```python
from build123d import *

# Parameters (mm, degrees)
MAIN_SKETCH_W        = 110
MAIN_SKETCH_H        = 72
MAIN_EXTRUSION_DEPTH = 6
MAIN_HOLE_SKETCH_R   = 1
MAIN_HOLE_SKETCH_R_2 = 0.9
MAIN_HOLE_DEPTH      = 7
EPIA_FIX_SKETCH_W    = 77
EPIA_FIX_SKETCH_H    = 40
EPIA_FIX_SKETCH_W_2  = 15
EPIA_FIX_SKETCH_H_2  = 8
EPIA_FIX_SKETCH_W_3  = 10
EPIA_FIX_SKETCH_W_4  = 8
EPIA_FIX_SKETCH_H_3  = 16
EPIA_FIX_DEPTH       = 4
FIX_SKETCH_R         = 1.35
FIX_HOLE_DEPTH       = 7


with BuildPart() as part:
    # Main-Sketch → Main-Extrusion (new body)
    with BuildSketch(Plane.XY):
        with Locations((55, 36)):
            Rectangle(MAIN_SKETCH_W, MAIN_SKETCH_H)
    extrude(amount=MAIN_EXTRUSION_DEPTH)

    # Main-Hole-Sketch → Main-Hole (cut, through all)
    with BuildSketch(Plane.XY.offset(6)):
        with Locations((7.5, 69.5)):
            Circle(MAIN_HOLE_SKETCH_R)
        with Locations((7.5, 2.5)):
            Circle(MAIN_HOLE_SKETCH_R_2)
        with Locations((102.5, 2.5)):
            Circle(MAIN_HOLE_SKETCH_R)
        with Locations((102.5, 69.5)):
            Circle(MAIN_HOLE_SKETCH_R)
    extrude(amount=-MAIN_HOLE_DEPTH, mode=Mode.SUBTRACT)

    # Epia-Fix-Sketch → Epia-Fix (cut)
    with BuildSketch(Plane.XY):
        with Locations((43.5, 27)):
            Rectangle(EPIA_FIX_SKETCH_W, EPIA_FIX_SKETCH_H)
        with Locations((32.5, 68)):
            Rectangle(EPIA_FIX_SKETCH_W_2, EPIA_FIX_SKETCH_H_2)
        with Locations((95, 68)):
            Rectangle(EPIA_FIX_SKETCH_W_3, EPIA_FIX_SKETCH_H_2)
        with Locations((98, 31)):
            Rectangle(EPIA_FIX_SKETCH_W_4, EPIA_FIX_SKETCH_H_3)
    extrude(amount=EPIA_FIX_DEPTH, mode=Mode.SUBTRACT)

    # Fix-Sketch → Fix-Hole (cut, through all)
    with BuildSketch(Plane.XY.offset(6)):
        with Locations((107, 69)):
            Circle(FIX_SKETCH_R)
        with Locations((107, 3)):
            Circle(FIX_SKETCH_R)
        with Locations((3, 69)):
            Circle(FIX_SKETCH_R)
        with Locations((3, 3)):
            Circle(FIX_SKETCH_R)
    extrude(amount=-FIX_HOLE_DEPTH, mode=Mode.SUBTRACT)


solid = part.part
```
For this review, take the finished solid that the model builds, in its own axes (mm). A direction names the side the tool comes from. Give positions to 0.01 mm unless a question says otherwise; leave off trailing zeros. Write each loop counter-clockwise with the first axis right and the second up, starting at its lowest first coordinate (ties: lowest second). Pieces come first, ordered by that corner, then holes. Notation, with made-up numbers: M 2,54.5 L 23,54.5 A11 cw 23,64.5 Z; hole C 13,-0.75 d11. An arc over 180 degrees is marked long. One line per item, written item: value.
1) Take a section at B-B, the plane y = 16. Write out the cut boundary in (x, z).
Results are:
outline: M 0,0 L 5,0 L 5,4 L 82,4 L 82,0 L 110,0 L 110,6 L 0,6 Z
2) Take a section at C-C, the plane z = 1.9. Count the separate pieces of the cut face and the enclosed holes in it, then the cut area to 3 significant figures.
Results are:
separate pieces: 1
enclosed holes: 10
area: 4,480 mm²
3) Take a section at D-D, the plane x = 32.5. Write out the cut boundary in (y, z).
Results are:
outline: M 0,0 L 7,0 L 7,4 L 47,4 L 47,0 L 64,0 L 64,4 L 72,4 L 72,6 L 0,6 Z
4) The part is to be moulded in two halves that separate along X. For faces 1 (the flat face through (54, 0, 3)), 2 (the flat face through (32, 64, 2)), 3 (the flat face through (110, 35, 3)), say which applies: +X half, -X half, draft (parallel to the pull), parting line (faces both ways), or undercut.
Results are:
face 1: draft
face 2: undercut
face 3: +X half
5) For line 1 (Y direction, x = 3, z = 2.4); line 2 (X direction, y = 20.5, z = 2.7); line 3 (Y direction, x = 7.5, z = 1.4), list the stretches that pass through material, from the lowest coordinate up. Write a range as from..to.
Results are:
line 1: y = 0..1.65, 4.35..67.65, 70.35..72
line 2: x = 0..5, 82..110
line 3: y = 0..1.6, 3.4..7, 47..68.5, 70.5..72
6) For faces 4 (the flat face through (25, 68, 2)), 5 (the flat face through (102, 31, 2)), 6 (the flat face through (66, 53, 0)), list the 3-axis set-ups (+Z, -Z, +X, -X, +Y, -Y) from which the entire face can be reached by the end or side of a thin tool; tool diameter is ignored.
Results are:
face 4: -Z, +Y
face 5: -Z
face 6: -Z, +X, -X, +Y, -Y
7) Take a section at A-A, the plane x = 107. Write out the cut boundary in (y, z), then the cut area to 3 significant figures.
Results are:
outline: M 0,0 L 1.65,0 L 1.65,6 L 0,6 Z; M 4.35,0 L 67.65,0 L 67.65,6 L 4.35,6 Z; M 70.35,0 L 72,0 L 72,6 L 70.35,6 Z
area: 400 mm²
8) For P1, Ø3, axis at x = 73, y = 20.5, coming from the -Z side; P2, Ø2.5, axis at x = 3, y = 69, coming from the -Z side; P3, Ø3, axis at y = 45, z = 4, coming from the -X side, all flat-tipped, find the tip position at first contact; note any pin that passes through.
Results are:
P1: stops at z = 4
P2: passes through
P3: stops at x = 0
